from build123d import *

# Parameters (mm, degrees)
F1_DEPTH = 7.62


with BuildPart() as f1:
    # F0 (on Front) → F1 (new body)
    with BuildSketch(Plane.XZ):
        with BuildLine():
            Line((1.8622589664, 6.0707900262), (0, 6.35))
            ThreePointArc((0, 6.35), (-6.35, 0), (0, -6.35))
            Line((0, -6.35), (1.8187823812, -6.0839568251))
            ThreePointArc((1.8187823812, -6.0839568251), (5.0927285477, -3.7929692775), (6.35, 0))
            ThreePointArc((6.35, 0), (5.1062630385, 3.7747288355), (1.8622589664, 6.0707900262))
        make_face()
        with BuildLine():
            ThreePointArc((4.4081076155, 0.5715), (4.4357673153, 0.2863447651), (4.445, 0))
            ThreePointArc((4.445, 0), (4.4357673153, -0.2863447651), (4.4081076155, -0.5715))
            ThreePointArc((4.4081076155, -0.5715), (3.1430896424, -3.1430896424), (0.5715, -4.4081076155))
            ThreePointArc((0.5715, -4.4081076155), (0, -4.445), (-0.5715, -4.4081076155))
            ThreePointArc((-0.5715, -4.4081076155), (-3.1430896424, -3.1430896424), (-4.4081076155, -0.5715))
            ThreePointArc((-4.4081076155, -0.5715), (-4.445, 0), (-4.4081076155, 0.5715))
            ThreePointArc((-4.4081076155, 0.5715), (-3.1430896424, 3.1430896424), (-0.5715, 4.4081076155))
            ThreePointArc((-0.5715, 4.4081076155), (0, 4.445), (0.5715, 4.4081076155))
            ThreePointArc((0.5715, 4.4081076155), (3.1430896424, 3.1430896424), (4.4081076155, 0.5715))
        make_face(mode=Mode.SUBTRACT)
        with BuildLine():
            ThreePointArc((1.8622589664, 6.0707900262), (0.9415368643, 6.2798095778), (0, 6.35))
            Line((0, 6.35), (1.8622589664, 6.0707900262))
        make_face()
        with BuildLine():
            Line((1.8187823812, -6.0839568251), (0, -6.35))
            ThreePointArc((0, -6.35), (0.9190685939, -6.2831371877), (1.8187823812, -6.0839568251))
        make_face()
        with BuildLine():
            Line((13.9979512441, 4.2512759929), (1.8622589664, 6.0707900262))
            ThreePointArc((1.8622589664, 6.0707900262), (5.1062630385, 3.7747288355), (6.35, 0))
            ThreePointArc((6.35, 0), (5.0927285477, -3.7929692775), (1.8187823812, -6.0839568251))
            Line((1.8187823812, -6.0839568251), (13.9979512441, -4.3024436627))
            add(Edge.make_bspline(
                [(12.9819512441, -4.3278436627), (13.3216856344, -4.3582096926), (13.6625330249, -4.3515071069), (13.9979512441, -4.3024436627)],
                knots=[0.9379354435, 0.9379354435, 0.9379354435, 0.9379354435, 1, 1, 1, 1], degree=3))
            add(Edge.make_bspline(
                [(11.8986046127, -4.1080734588), (12.2530212332, -4.2197633946), (12.616843509, -4.2952097206), (12.9819512441, -4.3278436627)],
                knots=[0.8712355441, 0.8712355441, 0.8712355441, 0.8712355441, 0.9379354435, 0.9379354435, 0.9379354435, 0.9379354435], degree=3))
            add(Edge.make_bspline(
                [(11.8973232208, 4.0530741781), (9.9551383056, 3.4340248692), (6.5706535126, -0.0030113398), (9.9231723965, -3.4855408669), (11.8986046127, -4.1080734588)],
                knots=[0.1307760808, 0.1307760808, 0.1307760808, 0.1307760808, 0.4994664947, 0.8712355441, 0.8712355441, 0.8712355441, 0.8712355441], degree=3))
            add(Edge.make_bspline(
                [(13.9979512441, 4.2512759929), (13.30745774, 4.3548022353), (12.5862245912, 4.2726536393), (11.8973232208, 4.0530741781)],
                knots=[0, 0, 0, 0, 0.1307760808, 0.1307760808, 0.1307760808, 0.1307760808], degree=3))
        make_face()
        with BuildLine():
            Line((13.9979512441, 3.6924759929), (13.9979512441, 4.2512759929))
            add(Edge.make_bspline(
                [(13.9979512441, 4.2512759929), (13.30745774, 4.3548022353), (12.5862245912, 4.2726536393), (11.8973232208, 4.0530741781)],
                knots=[0, 0, 0, 0, 0.1307760808, 0.1307760808, 0.1307760808, 0.1307760808], degree=3))
            Line((11.8973232208, 4.0530741781), (12.9819512441, 3.6924759929))
            Line((12.9819512441, 3.6924759929), (13.9979512441, 3.6924759929))
        make_face()
        with BuildLine():
            add(Edge.make_bspline(
                [(12.9819512441, -4.3278436627), (13.3216856344, -4.3582096926), (13.6625330249, -4.3515071069), (13.9979512441, -4.3024436627)],
                knots=[0.9379354435, 0.9379354435, 0.9379354435, 0.9379354435, 1, 1, 1, 1], degree=3))
            Line((13.9979512441, -4.3024436627), (13.9979512441, -3.7436436627))
            Line((13.9979512441, -3.7436436627), (12.9819512441, -3.7436436627))
            Line((12.9819512441, -3.7436436627), (11.8986046127, -4.1080734588))
            add(Edge.make_bspline(
                [(11.8986046127, -4.1080734588), (12.2530212332, -4.2197633946), (12.616843509, -4.2952097206), (12.9819512441, -4.3278436627)],
                knots=[0.8712355441, 0.8712355441, 0.8712355441, 0.8712355441, 0.9379354435, 0.9379354435, 0.9379354435, 0.9379354435], degree=3))
        make_face()
        with BuildLine():
            ThreePointArc((4.4081076155, -0.5715), (4.4357673153, -0.2863447651), (4.445, 0))
            ThreePointArc((4.445, 0), (4.4357673153, 0.2863447651), (4.4081076155, 0.5715))
            Line((4.4081076155, 0.5715), (3.8493076155, 0.5715))
            Line((3.8493076155, 0.5715), (3.8493076155, -0.5715))
            Line((3.8493076155, -0.5715), (4.4081076155, -0.5715))
        make_face()
        with BuildLine():
            ThreePointArc((-0.5715, -4.4081076155), (0, -4.445), (0.5715, -4.4081076155))
            Line((0.5715, -4.4081076155), (0.5715, -3.8493076155))
            Line((0.5715, -3.8493076155), (-0.5715, -3.8493076155))
            Line((-0.5715, -3.8493076155), (-0.5715, -4.4081076155))
        make_face()
        with BuildLine():
            Line((-3.8493076155, 0.5715), (-4.4081076155, 0.5715))
            ThreePointArc((-4.4081076155, 0.5715), (-4.445, 0), (-4.4081076155, -0.5715))
            Line((-4.4081076155, -0.5715), (-3.8493076155, -0.5715))
            Line((-3.8493076155, -0.5715), (-3.8493076155, 0.5715))
        make_face()
        with BuildLine():
            Line((0.5715, 3.8493076155), (0.5715, 4.4081076155))
            ThreePointArc((0.5715, 4.4081076155), (0, 4.445), (-0.5715, 4.4081076155))
            Line((-0.5715, 4.4081076155), (-0.5715, 3.8493076155))
            Line((-0.5715, 3.8493076155), (0.5715, 3.8493076155))
        make_face()
    extrude(amount=F1_DEPTH)


solid = f1.part
Here's how the part is built. I have some questions about the finished solid (model axes, mm). A direction names the side the tool comes from. Coordinates: 2 decimals unless noted, no trailing zeros.
1. If we mould it in two halves opening along Z, with no side actions, what happens to faces 4 (the flat face through (6, -7.62, 0)), 5 (the flat face through (8.015, -3.757, 5.148)), 6 (the cylindrical face through (-3.172, -3.757, 3.114)), 7 (the flat face through (12.448, -3.757, -3.923))? For each: pulls with the +Z half, pulls with the -Z half, needs draft (parallel to the pull), parting line crosses it, or undercut.
2. I need wall thicknesses on L1, parallel to X at y = -6.25, z = 0 (3 decimals); L2, parallel to Z at x = 11, y = -6.5; L3, parallel to X at y = -3.75, z = -0.75. Which ranges of each line are inside material? Lowest first, please.
3. For faces 1 (the flat face through (13.5, -3.8, 3.692)), 2 (the flat face through (12.432, -3.757, 3.875)), 3 (the flat face through (6, 0, 0)), which set-ups out of +Z, -Z, +X, -X, +Y, -Y let a thin tool reach every point of the face, with its end or its side?
4. For P1, Ø1, axis at y = -3.5, z = -2.5, coming from the +X side; P2, Ø0.6, axis at y = -3.5, z = 0, coming from the +X side; P3, Ø2, axis at x = 8, y = -1.5, coming from the +Z side, each with a flat end and sliding along its axis, tell me the tip position at first contact or that it passes through.
Taken from the geometry:
1. face 4: needs draft
1. face 5: pulls with the +Z half
1. face 6: undercut
1. face 7: undercut
2. L1: x = -6.35 to -3.849, 3.849 to 8.255
2. L2: z = -4.74 to -3.74, 3.68 to 4.7
2. L3: x = -6.31 to -4.38, 4.38 to 8.35
3. face 1: +X, +Y, -Y
3. face 2: +Y, -Y
3. face 3: +Z, -Z, +X, -X, +Y
4. P1: stops at x = 9.88
4. P2: stops at x = 8.27
4. P3: stops at z = 5.3
